Study the drawing (mm; zero at the part's minimum x, y, z) and answer. Give positions to 0.01 mm unless a question says otherwise; leave off trailing zeros. Order: outer loops, then holes, each group sorted by start corner. A loop starts at its lowest first (then second) coordinate and runs counter-clockwise, first axis right, second up. Notation, with made-up numbers: (30.5, 13.5) - (87.5, 13.5) arc R31 ccw to (87.5, 48.5) - close; hole circle Ø3 at (64.25, 44.5). An arc over 180 degrees is marked (long way). Return JSON: item names as keys, results as strings.
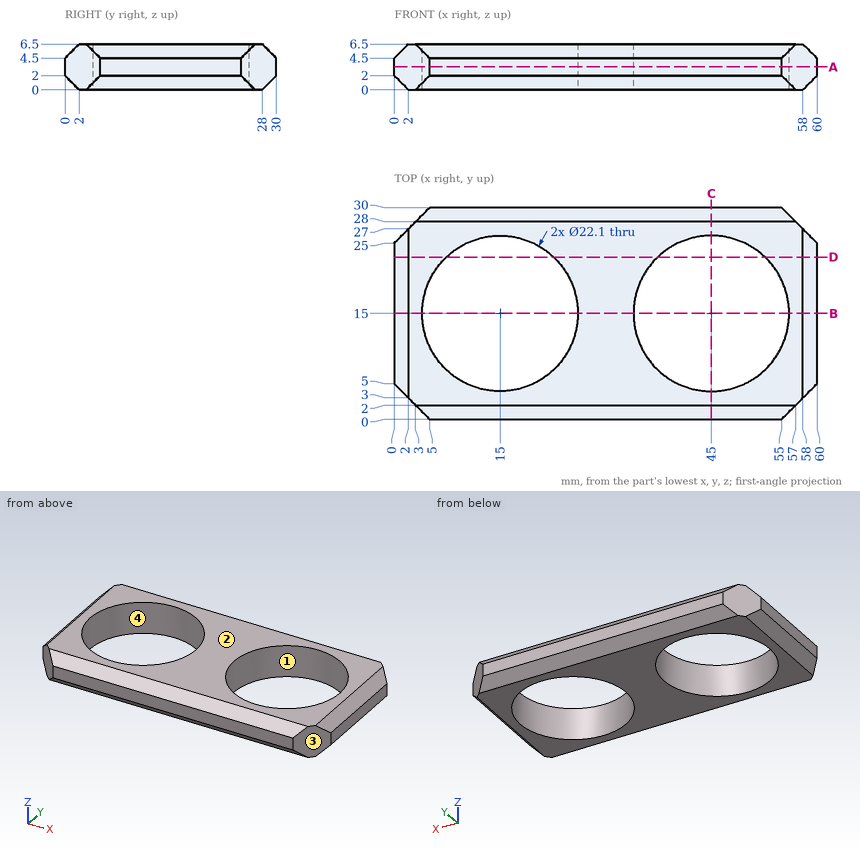
Q1. A cutting plane is placed at D-D (y = 23). Write down the section's boundary in (x, z).
Values:
{"outline": "(0, 2) - (2, 0) - (7.38, 0) - (7.38, 6.5) - (2, 6.5) - (0, 4.5) - close; (22.62, 0) - (37.38, 0) - (37.38, 6.5) - (22.62, 6.5) - close; (52.62, 0) - (58, 0) - (60, 2) - (60, 4.5) - (58, 6.5) - (52.62, 6.5) - close"}
Q2. A cutting plane is placed at B-B (y = 15). Write down the section's boundary in (x, z).
Values:
{"outline": "(0, 2) - (2, 0) - (3.95, 0) - (3.95, 6.5) - (2, 6.5) - (0, 4.5) - close; (26.05, 0) - (33.95, 0) - (33.95, 6.5) - (26.05, 6.5) - close; (56.05, 0) - (58, 0) - (60, 2) - (60, 4.5) - (58, 6.5) - (56.05, 6.5) - close"}
Q3. A cutting plane is placed at C-C (x = 45). Write down the section's boundary in (y, z), and give its area (4 significant figures).
Values:
{"outline": "(0, 2) - (2, 0) - (3.95, 0) - (3.95, 6.5) - (2, 6.5) - (0, 4.5) - close; (26.05, 0) - (28, 0) - (30, 2) - (30, 4.5) - (28, 6.5) - (26.05, 6.5) - close", "area": "43.35 mm²"}
Q4. Consider L1, parallel to X at y = 14.25, z = 4.25; L2, parallel to X at y = 10, z = 5; L3, parallel to Y at x = 45, z = 2.75. Determine where each line is inside the solid, lowest interval first.
Values:
{"L1": "x = 0 to 3.98, 26.02 to 33.98, 56.02 to 60", "L2": "x = 0.5 to 5.15, 24.85 to 35.15, 54.85 to 59.5", "L3": "y = 0 to 3.95, 26.05 to 30"}
Q5. A cutting plane is placed at A-A (z = 3.25). Write down the section's boundary in (x, y), and give its area (3 significant figures).
Values:
{"outline": "(0, 5) - (5, 0) - (55, 0) - (60, 5) - (60, 25) - (55, 30) - (5, 30) - (0, 25) - close; hole circle Ø22.1 at (15, 15); hole circle Ø22.1 at (45, 15)", "area": "983 mm²"}
Q6. Given pin 1 (17.5 mm diameter, centred on x = 15, y = 15, fed in from +Z); pin 2 (1 mm diameter, centred on y = 27, z = 5.5, fed in from -X), each flat-ended and moving along its own axis, determine where each tip first touches the part or whether it passes through.
Values:
{"pin 1": "passes through", "pin 2": "stops at x = 1.5"}
Q7. Determine the mould class of the marked faces 1, 2, 3 and 4 for opening direction X: released by +X, released by -X, zero draft, split by the parting line, or undercut.
Values:
{"face 1": "undercut", "face 2": "zero draft", "face 3": "released by +X", "face 4": "undercut"}
